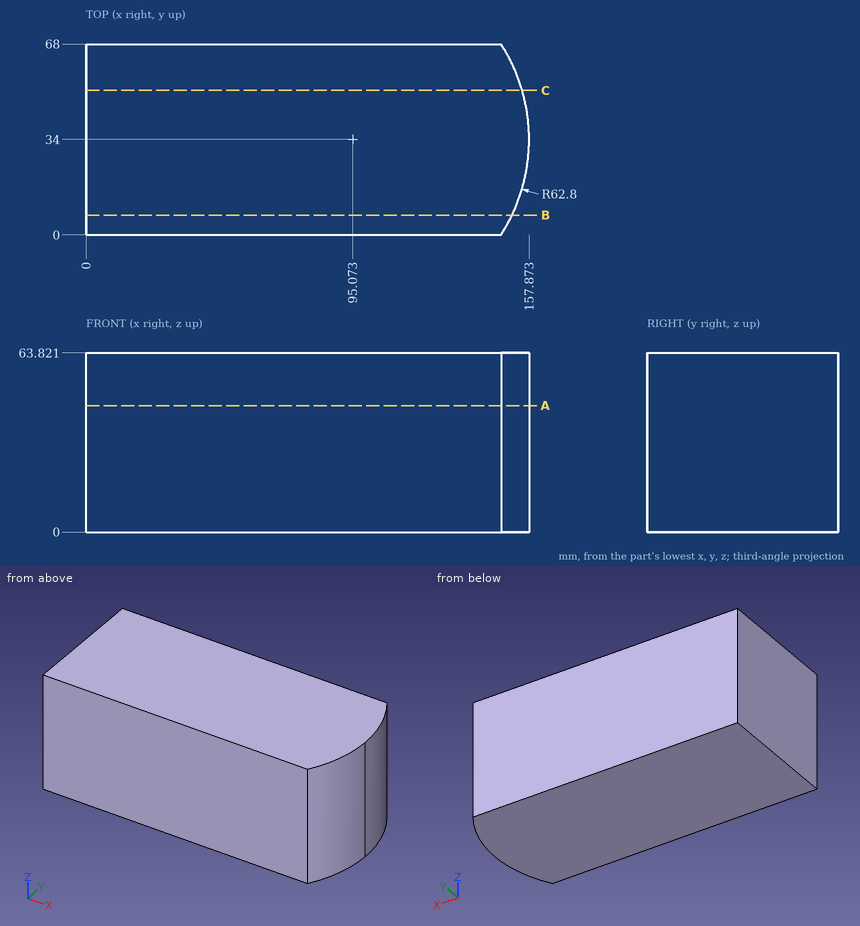
Print and shaded views of the part. All mm, measured from the part's lowest x, y and z. Round coordinates to 2 decimals unless told otherwise and drop trailing zeros. Write each loop counter-clockwise with the first axis right and the second up, starting at its lowest first coordinate (ties: lowest second). Pieces come first, ordered by that corner, then holes. Notation, with made-up numbers: (56.5, -6.5) - (90.5, -6.5) arc R24 ccw to (90.5, 11.5) - close; hole circle Ø6 at (57.25, 80.25). An arc over 180 degrees is marked (long way). Use CSV: the item, a comma, the result in double quotes. Start each with the question number.
Item 1: Pin check, flat tips, straight feed: P1, Ø5, axis at y = 15.5, z = 30, coming from the -X side; P2, Ø6, axis at y = 58, z = 48, coming from the +X side; P3, Ø10, axis at y = 8.5, z = 49.5, coming from the +X side; P4, Ø2, axis at y = 54.5, z = 50.5, coming from the +X side. Stop position of each tip, or through.
Item 2: Band-saw the part on C-C (y = 51.5). Write the cut outline in (x, z), and give its area (3 significant figures).
Item 3: Drill centre lines: L1, parallel to X at y = 21.5, z = 42; L2, parallel to X at y = 60.5, z = 28.5. Where is each one in solid material? Low to high. Write a range as [from, to].
Item 4: Band-saw the part on B-B (y = 7). Write the cut outline in (x, z).
Item 5: Band-saw the part on A-A (z = 45). Write the cut outline in (x, y).
Checked values:
1,P1,"stops at x = 0"
1,P2,"stops at x = 154.26"
1,P3,"stops at x = 154.43"
1,P4,"stops at x = 154.77"
2,outline,"(0, 0) - (155.39, 0) - (155.39, 63.82) - (0, 63.82) - close"
2,area,"9,920 mm²"
3,L1,"x = [0, 156.62]"
3,L2,"x = [0, 152.01]"
4,outline,"(0, 0) - (151.77, 0) - (151.77, 63.82) - (0, 63.82) - close"
5,outline,"(0, 0) - (147.87, 0) arc R62.8 ccw to (157.87, 34) arc R62.8 ccw to (147.87, 68) - (0, 68) - close"
